from build123d import *

# Parameters (mm, degrees)
F0_W     = 160
F0_H     = 68
F1_DEPTH = 12
F3_DEPTH = 12
F4_W     = 6
F4_H     = 68
F5_DEPTH = 12


with BuildPart() as f1:
    # F0 (on Front) → F1 (new body)
    with BuildSketch(Plane.XZ):
        Rectangle(F0_W, F0_H)
    extrude(amount=F1_DEPTH)

    # F2 (on face) → F3 (cut)
    with BuildSketch(Plane.YZ.offset(80)):
        Polygon((-6, 22), (-6, 34), (-12, 34), (-12, -34), (-6, -34), align=None)
    extrude(amount=-F3_DEPTH, mode=Mode.SUBTRACT)

    # F4 (on face) → F5 (cut)
    with BuildSketch(Plane(origin=(-80, 0, 0), x_dir=(0, -1, 0), z_dir=(-1, 0, 0))):
        with Locations((9, 0)):
            Rectangle(F4_W, F4_H)
    extrude(amount=-F5_DEPTH, mode=Mode.SUBTRACT)


solid = f1.part
Design review of the part built by this model. Coordinates are the model's own, in mm. A direction names the side the tool comes from. Give positions to 0.01 mm unless a question says otherwise; leave off trailing zeros. Write each loop counter-clockwise with the first axis right and the second up, starting at its lowest first coordinate (ties: lowest second). Pieces come first, ordered by that corner, then holes. Notation, with made-up numbers: M 85.25,60.25 L 128.25,60.25 A17 ccw 128.25,73.25 Z; hole C -29.5,55.5 d11. An arc over 180 degrees is marked long. Return JSON: item names as keys, results as strings. Group by question number.
Item 1: Tool access review of faces 1 (the flat face through (-74, -6, 0)), 2 (the flat face through (-1, -12, 0)), 3 (the flat face through (74, -6, 0)): name each direction out of +Z, -Z, +X, -X, +Y, -Y from which nothing blocks a thin tool from reaching the whole face with its end or side.
Item 2: Take a section at A-A (z = -6). Give the boundary of the cut face in (x, y).
Item 3: Take a section at B-B (x = 70). Give the boundary of the cut face in (y, z).
Item 4: Wall thickness on line 1 along X through (y, z) = (-8, -6.5); line 2 along Y through (x, z) = (-72, 17): over which ranges is each line inside the solid? List them lowest first.
Item 5: Clearance check with flat-ended pins moving along their axes: pin 1 Ø3 at (y, z) = (-9, -2) entering from -X; pin 2 Ø5 at (y, z) = (-9.5, 12) entering from +X; pin 3 Ø13 at (x, z) = (-77, -13.5) entering from -Y. State where each tip first meets the part, or that it passes through.
Return value:
{
 "1": {"face 1": "+Z, -Z, -X, -Y", "face 2": "+Z, -Z, +X, -X, -Y", "face 3": "+Z, -Z, +X, -Y"},
 "2": {"outline": "M -80,-6 L -68,-6 L -68,-12 L 68,-12 L 68,-6 L 80,-6 L 80,0 L -80,0 Z"},
 "3": {"outline": "M -6,-34 L 0,-34 L 0,34 L -6,34 Z"},
 "4": {"line 1": "x = -68 to 68", "line 2": "y = -6 to 0"},
 "5": {"pin 1": "stops at x = -68", "pin 2": "stops at x = 68", "pin 3": "stops at y = -6"}
}
